Autodesk Inventor part; units mm, degrees
ref_plane "Plan de construction2" through (6, 0, -4.9) normal (0, 0, -1) x (-1, 0, 0)
ref_plane "YZ Plane" through (0, 0, 0) normal (1, 0, 0) x (0, 1, 0)
ref_plane "XZ Plane" through (0, 0, 0) normal (0, 1, 0) x (-1, 0, 0)
sketch "Sketch1" plane through (0, 0, 0) normal (0, 0, 1) x (1, 0, 0)
  line L0 (0, 0) -> (34, 0) construction
  line L1 (0, 0) -> (0, 4.9) construction
  line L2 (0, 4.9) -> (12, 4.9)
  line L3 (12, 4.9) -> (12, 2.5)
  line L4 (12, 2.5) -> (34, 2.5)
  line L5 (34, 2.5) -> (34, 0) construction
  line L6 (0, 4.9) -> (0, 2.45)
  line L7 (0, 2.45) -> (6, 2.45)
  line L8 (6, 2.45) -> (6, 0)
  line L9 (34, 2.5) -> (34, 0)
  line L10 (6, 0) -> (34, 0)
  dimension "d0" = 34
  dimension "d3" = 12
  dimension "d4" = 9.8
  dimension "d5" = 4.9
  dimension "d6" = 6
  dimension "d7" = 5
revolve "Révolution1" add sketch "Sketch1" angle 360 about axis through (6, 0, 0) along (1, 0, 0)
sketch "Esquisse2" plane through (34, 0, 0) normal (1, 0, 0) x (0, 0, -1)
  circle A0 centre (0, 0) radius 2.5 construction
  line L0 (-1.5, -2) -> (-1.5, 2)
  arc A1 (-1.5, 2) -> (-1.5, -2) centre (0, 0) ccw
  dimension "d9" = 1.5
extrude "Extrusion1" cut sketch "Esquisse2" against normal blind 5
ref_plane "Plan de construction2" through (6, 0, -4.9) normal (0, 0, -1) x (-1, 0, 0)
ref_plane "Plan de construction1" through (6, 0, 4.9) normal (0, 0, 1) x (1, 0, 0)
sketch "Esquisse4" plane through (6, 0, -4.9) normal (0, 0, -1) x (-1, 0, 0)
  line L0 (6, 4.9) -> (6, -4.9) construction
  point P0 (6, 0)
  point P1 (4, 0)
  dimension "d20" = 2
hole "Perçage2" at (2, 0, -4.9) direction (0, 0, 1) diameter 1.567 depth 5 tip angle 118 countersink diameter 2.2 countersink angle 90
properties part number "M000" material "Acier"
Source: CAD feature listing. Evaluate the final solid. Frame: model axes, mm. A direction names the side the tool comes from. Round coordinates to 2 decimals unless told otherwise and drop trailing zeros. Loops run counter-clockwise (first coordinate to the right, second up) from the corner with the lowest first, then second, coordinate; pieces in that order, holes last. Notation, with made-up numbers: (-39, 16.25) - (13, 16.25) arc R33 ccw to (13, 51.25) - close; hole circle Ø11 at (85, -33.5). An arc over 180 degrees is marked (long way). Write item = value, one per line. Start each with the question number.
Item 1: First-contact query: pin 1 Ø3 at (x, y) = (32, 0.5) entering from +Z; pin 2 Ø2 at (x, z) = (14.5, 2) entering from -Y; pin 3 Ø5 at (y, z) = (-1.5, -1.5) entering from -X; pin 4 Ø1 at (x, y) = (13.5, 1) entering from +Z. Flat tips, straight axial feed; report the tip coordinate or a pass-through.
Item 2: Reachability of faces 4 (the face through (2.3, 0.724, -3.436)), 5 (the face through (23.15, -0.54, -2.44)), 6 (the face through (6, 0, 0)) from +Z, -Z, +X, -X, +Y, -Y: full face, straight path, thin tool, end or side. Return the list, or none.
Item 3: Section query A-A on y = 0. Output: boundary loops of the cut face in (x, z).
Item 4: Section query D-D on z = -3.5. Output: boundary loops of the cut face in (x, y).
Item 5: Section query C-C on x = 16. Output: boundary loops of the cut face in (y, z).
Item 6: Material intervals for line 1 (Y direction, x = 24, z = 1.5); line 2 (X direction, y = -2.25, z = -3.75); line 3 (Z direction, x = 8.5, y = 0.25), sorted ascending.
Item 7: Section query B-B on z = 0. Output: boundary loops of the cut face in (x, y).
Item 8: Mould query, pull axis Z, two halves, no side actions, for faces 1 (the face through (34, 0, 0)), 2 (the face through (6.084, -1.062, -4.783)), 3 (the face through (3.042, 1.317, 2.066)). Classes: released by +Z, released by -Z, zero draft, split by the parting line, or undercut.
Results list:
q1.pin_1 = 1.5
q1.pin_2 = -2.29
q1.pin_3 = 0
q1.pin_4 = 2.45
q2.face_4 = -Z
q2.face_5 = +X
q2.face_6 = -X
q3.outline = (0, -4.9) - (0.9, -4.9) - (1.22, -4.58) - (1.22, -2.45) - (0, -2.45) - close; (0, 2.45) - (6, 2.45) - (6, -2.45) - (2.78, -2.45) - (2.78, -4.58) - (3.1, -4.9) - (12, -4.9) - (12, -2.5) - (34, -2.5) - (34, 1.5) - (29, 1.5) - (29, 2.5) - (12, 2.5) - (12, 4.9) - (0, 4.9) - close
q4.outline = (0, -3.43) - (12, -3.43) - (12, 3.43) - (0, 3.43) - close; hole circle Ø1.57 at (2, 0)
q5.outline = circle Ø5 at (0, 0)
q6.line_1 = -2 to 2
q6.line_2 = 0 to 12
q6.line_3 = -4.89 to 4.89
q7.outline = (0, -4.9) - (12, -4.9) - (12, -2.5) - (34, -2.5) - (34, 2.5) - (12, 2.5) - (12, 4.9) - (0, 4.9) - (0, 2.45) - (6, 2.45) - (6, -2.45) - (0, -2.45) - close
q8.face_1 = zero draft
q8.face_2 = split by the parting line
q8.face_3 = undercut
